Can you work these out from the model? Positions are in its coordinate system, mm. Face numbers are marked on the shaded views. A direction names the side the tool comes from. Coordinates: 2 decimals unless noted, no trailing zeros. Loops run counter-clockwise (first coordinate to the right, second up) from the corner with the lowest first, then second, coordinate; pieces in that order, holes last.
```python
from build123d import *

# Parameters (mm, degrees)
F0_R     = 1.8
F1_DEPTH = 14
F2_W     = 5.5
F2_H     = 4.0708386075
F2_H_2   = 4.9094793208
F3_DEPTH = 5
F4_W     = 11
F4_H     = 7.5
F5_DEPTH = 12
F6_R     = 0.2312376478
F7_W     = 8.2372972146
F7_H     = 9.0102642961
F8_DEPTH = 5


# Not quite as in the source:
# - a feature names something its author has since deleted; it is built from what else it names


with BuildPart() as f1:
    # F0 (on Right) → F1 (new body)
    with BuildSketch(Plane.YZ):
        with BuildLine():
            Line((-9.1132364464, -5), (0, -5))
            Line((0, -5), (0, 2.1922827341))
            Line((0, 2.1922827341), (1.4037047395, 3.5753551798))
            ThreePointArc((1.4037047395, 3.5753551798), (7.0067613017, 4.6816844814), (10.2298574217, -0.0331706346))
            Line((10.2298574217, -0.0331706346), (10.3112826954, -4.9419746769))
            Line((10.3112826954, -4.9419746769), (12.3110075686, -4.9088040424))
            Line((12.3110075686, -4.9088040424), (12.2295822948, 0))
            ThreePointArc((12.2295822948, 0), (7.7636365241, 6.5329380451), (0, 5))
            Line((0, 5), (-9.1132364464, 5))
            ThreePointArc((-9.1132364464, 5), (-14.1132364464, 0), (-9.1132364464, -5))
        make_face()
        with Locations((-9.5687768728, 0)):
            Circle(F0_R, mode=Mode.SUBTRACT)
    extrude(amount=F1_DEPTH)

    # F2 (on face) → F3 (cut)
    with BuildSketch(Plane(origin=(0, 12.2262182699, 0.2028036077), x_dir=(-1, 0, 0), z_dir=(0, 0.9998624542, 0.0165853176))):
        with Locations((-7, 1.8325877974)):
            Rectangle(F2_W, F2_H)
        with Locations((-7, -2.6575711668)):
            Rectangle(F2_W, F2_H_2)
    extrude(amount=-F3_DEPTH, mode=Mode.SUBTRACT)

    # F4 (on face) → F5 (cut)
    with BuildSketch(Plane(origin=(0, 0, -5), x_dir=(1, 0, 0), z_dir=(0, 0, -1))):
        with Locations((7, 5.3632364464)):
            Rectangle(F4_W, F4_H)
        with Locations((7, 12.8632364464)):
            Rectangle(F4_W, F4_H)
    extrude(amount=-F5_DEPTH, mode=Mode.SUBTRACT)

    # F6
    f6_edges = [f1.edges().sort_by_distance(p)[0] for p in [
        (1.5, -11.368777, 0),
        (12.5, -11.368777, 0),
        (0, -11.368777, 0),
        (14, -11.368777, 0),
        (7, 0, 2.192283),
        (12.5, -5.363236, -5),
        (1.5, -5.363236, -5),
        (12.5, -14.113236, 0),
        (12.5, -5.363236, 5),
        (1.5, -5.363236, 5),
        (1.5, -14.113236, 0),
    ]]
    fillet(f6_edges, radius=F6_R)

    # F7 (on face) → F8 (cut)
    with BuildSketch(Plane.XZ.offset(1.6132364464)):
        with Locations((7, -0.494867852)):
            Rectangle(F7_W, F7_H)
    extrude(amount=-F8_DEPTH, mode=Mode.SUBTRACT)


with BuildPart() as f9_1:
    # F9: copy of F1
    add(f1.part)


with BuildPart() as f11_1:
    # F11: copy of F1
    add(f1.part)


solid = f1.part
```
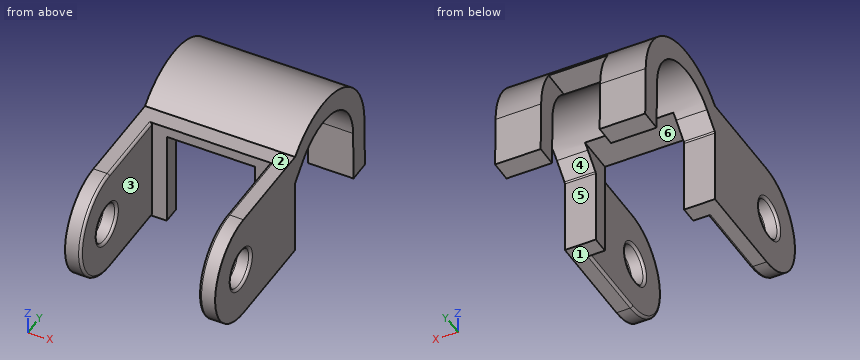
Item 1: Suppose I cut it at D-D, the plane z = 5.5. Please give me the cut outline in (x, y), plus the area to 3 significant figures.
Results are:
outline: (0, 0.56) - (14, 0.56) - (14, 9.52) - (0, 9.52) - close
area: 125 mm2
Item 2: On a 3-axis mill with a long thin cutter (end or side, diameter ignored), from which of +Z, -Z, +X, -X, +Y, -Y can I reach the whole of each face in a straight line? I mean the marked faces 1, 2, 3 and 4. Say none if no direction works.
Results are:
face 1: -Z, +X, -X, +Y, -Y
face 2: +Z, +X, -X, -Y
face 3: +Z, -Z, -Y
face 4: -Z, +X, -X
Item 3: Suppose I cut it at A-A, the plane x = 11.5. Please give me the cut outline in (y, z).
Results are:
outline: (-1.61, -5) - (0, -5) - (0, 2.1) arc R0.23 cw to (0.07, 2.26) - (1.4, 3.58) arc R5.19 cw to (10.23, -0.03) - (10.31, -4.94) - (12.31, -4.91) - (12.23, 0) arc R7.19 ccw to (0, 5) - (-1.61, 5) - close
Item 4: I need wall thicknesses on line 1 along Y through (x, z) = (12.25, -0.25); line 2 along X through (y, z) = (-3, 0.5); line 3 along Y through (x, z) = (13, 1). Which ranges of each line are inside material? Lowest first, please.
Results are:
line 1: y = -1.61 to 0, 10.23 to 12.23
line 2: x = 0 to 1.5, 12.5 to 14
line 3: y = -14.01 to -11.07, -8.07 to 0, 10.11 to 12.14
Item 5: I'm going to push flat-ended pins straight in: P1, Ø0.9, axis at x = 13, z = -1, coming from the +Y side; P2, Ø5, axis at x = 11.5, y = 8, coming from the -Z side; P3, Ø0.9, axis at x = 1.5, z = -0.5, coming from the +Y side. Where does each tip first touch, or does it pass through?
Results are:
P1: stops at y = 12.25
P2: stops at z = -4.94
P3: stops at y = 12.25
Item 6: We'd pull the mould along Y, two halves only. Please class the marked faces 5 and 6: +Y half, -Y half, draft (parallel to the pull), parting line (faces both ways), or undercut.
Results are:
face 5: undercut
face 6: draft
Item 7: Suppose I cut it at B-B, the plane z = 1.5. Count the separate pieces of the cut face and the enclosed holes in it, plus the area to 3 significant figures.
Results are:
separate pieces: 6
enclosed holes: 0
area: 57.6 mm2
